from build123d import *

# Parameters (mm, degrees)
F0_W      = 6.35
F0_H      = 6.35
F1_DEPTH  = 3.81
F2_R      = 2.3894248051
F3_DEPTH  = 25.4
F8_R      = 0.2232162281
F9_DEPTH  = 25.4
F10_R     = 2.7317429941
F11_DEPTH = 3.4770822
F12_W     = 5.8086237404
F12_H     = 6.0867127031
F13_DEPTH = 25.4


with BuildPart() as f1:
    # F0 (on Top) → F1 (new body)
    with BuildSketch(Plane.XY):
        with Locations((2.5444868952, -10.8615327454)):
            Rectangle(F0_W, F0_H)
    extrude(amount=F1_DEPTH)

    # F2 (on face) → F3 (join)
    with BuildSketch(Plane.XY.offset(3.81)):
        with Locations((2.5444868952, -10.8615327454)):
            Circle(F2_R)
    extrude(amount=F3_DEPTH)


with BuildPart() as f1_1:
    # F4: moved
    add(f1.part.moved(Location((-2.4892, 10.8204, 0))))

    # F5 (on Front) → F6 (revolve)
    with BuildSketch(Plane.XZ):
        with BuildLine():
            Line((3.715344239, 29.1360206902), (2.3982734419, 29.1360206902))
            Line((2.3982734419, 29.1360206902), (2.3982734419, 25.658948347))
            Line((2.3982734419, 25.658948347), (3.715344239, 25.658948347))
            ThreePointArc((3.715344239, 25.658948347), (3.8481047551, 26.626173701), (4.5479801483, 27.3068532688))
            Line((4.5479801483, 27.3068532688), (4.5479801483, 29.1360206902))
            Line((4.5479801483, 29.1360206902), (3.715344239, 29.1360206902))
        make_face()
    revolve(axis=Axis((0.0552868952, -0.0411327454, 29.21), (0, 0, 1)))


with BuildPart() as f1_2:
    # F7: moved
    add(f1_1.part.moved(Location((-0.0508, 0.0508, 0))))

    # F8 (on face) → F9 (cut)
    with BuildSketch(Plane.XY.offset(29.21)):
        with BuildLine():
            ThreePointArc((0.2196997185, 2.5085243013), (-0.06466925, 2.7232003988), (-0.1932256967, 2.3908981612))
            ThreePointArc((-0.1932256967, 2.3908981612), (-0.0028015905, 2.2853092181), (0.1869422498, 2.3921157731))
            ThreePointArc((0.1869422498, 2.3921157731), (0.2113543474, 2.4480594413), (0.2196997185, 2.5085243013))
        make_face()
        with Locations((-1.4773185054, 2.027371838)):
            Circle(F8_R)
        with Locations((-2.3868350443, 0.7718322405)):
            Circle(F8_R)
        with Locations((-2.3846617218, -0.7785210393)):
            Circle(F8_R)
        with Locations((-1.4716286733, -2.031505743)):
            Circle(F8_R)
        with Locations((0.0035165096, -2.5085243013)):
            Circle(F8_R)
        with Locations((1.4773185054, -2.027371838)):
            Circle(F8_R)
        with Locations((2.3868350443, -0.7718322405)):
            Circle(F8_R)
        with Locations((2.3846617218, 0.7785210393)):
            Circle(F8_R)
        with Locations((1.4716286733, 2.031505743)):
            Circle(F8_R)
    extrude(amount=-F9_DEPTH, mode=Mode.SUBTRACT)

    # F10 (on face) → F11 (join)
    with BuildSketch(Plane.XY.offset(29.1360206902)):
        Circle(F10_R)
    extrude(amount=-F11_DEPTH)

    # F12 (on face) → F13 (cut)
    with BuildSketch(Plane.XY.offset(29.1360206902)):
        with Locations((0.0104332576, 0.1239965204)):
            Rectangle(F12_W, F12_H)
    extrude(amount=F13_DEPTH, mode=Mode.SUBTRACT)


solid = f1_2.part
Model file for the job. Use its own axes, mm. A direction names the side the tool comes from. Round coordinates to 2 decimals unless told otherwise and drop trailing zeros. Loops run counter-clockwise (first coordinate to the right, second up) from the corner with the lowest first, then second, coordinate; pieces in that order, holes last. Notation, with made-up numbers: (15.5, 75.25) - (62.5, 75.25) arc R15 cw to (62.5, 93.25) - close; hole circle Ø4 at (-20.75, 81). An arc over 180 degrees is marked (long way). Write each question's results on one line, items separated by ' | '.
(1) Saw through at B-B, the plane z = 3. List the corners of the cut face in (x, y), then the cut area to 3 significant figures.
Answer below:
outline: (-3.17, -3.17) - (3.18, -3.17) - (3.18, 3.18) - (-3.17, 3.18) - close | area: 40.3 mm^2
(2) Wall check: L1, parallel to Z at x = -2.75, y = 1.5; L2, parallel to Y at x = -1.5, z = 8.75; L3, parallel to Y at x = -0.25, z = 10.5. Give the ranges that are in metal, low to high.
Answer below:
L1: z = 0 to 3.81, 25.66 to 29.14 | L2: y = -1.81 to 1.81 | L3: y = -2.37 to 2.39
(3) Mould opens along Z. For faces 6 (the cylindrical face through (-0.74, -2.26, 14.58)), 7 (the flat face through (-3.171, 0, 2)), 8 (the flat face through (0, 0, 0)) say: released by +Z, released by -Z, zero draft, split by the parting line, or undercut.
Answer below:
face 6: undercut | face 7: zero draft | face 8: released by -Z
(4) Pin check, flat tips, straight feed: pin 1 (1.1 mm diameter, centred on x = 1, z = 3, fed in from +Y); pin 2 (2 mm diameter, centred on x = -3, z = 18.5, fed in from -Y); pin 3 (5 mm diameter, centred on x = 2, z = 15, fed in from -Y). Stop position of each tip, or through.
Answer below:
pin 1: stops at y = 3.18 | pin 2: stops at y = -1.29 | pin 3: stops at y = -2.37
(5) 3-axis set-ups, long thin cutter, end or side, ignore diameter. For faces 1 (the cylindrical face through (0.75, 2.28, 14.58)), 2 (the cylindrical face through (0.731, -2.267, 14.582)), 3 (the flat face through (0, -3.165, 2)), 4 (the flat face through (-1.5, 2.2, 3.81)), 5 (the cylindrical face through (-1.928, -1.396, 14.582)): which of +Z, -Z, +X, -X, +Y, -Y reach the whole face in a straight line?
Answer below:
face 1: +X, +Y | face 2: +X, -Y | face 3: -Z, +X, -X, -Y | face 4: none | face 5: -X, -Y
(6) Saw through at A-A, the plane z = 14. List the corners of the cut face in (x, y), then the cut area to 3 significant figures.
Answer below:
outline: (-2.32, 0.56) arc R2.39 ccw to (-2.31, -0.57) arc R0.22 cw to (-2.2, -0.91) arc R2.39 ccw to (-1.54, -1.82) arc R0.22 cw to (-1.25, -2.02) arc R2.39 ccw to (-0.17, -2.37) arc R0.22 cw to (0.18, -2.37) arc R2.39 ccw to (1.25, -2.03) arc R0.22 cw to (1.55, -1.82) arc R2.39 ccw to (2.21, -0.91) arc R0.22 cw to (2.33, -0.56) arc R2.39 ccw to (2.33, 0.56) arc R0.22 cw to (2.21, 0.92) arc R2.39 ccw to (1.56, 1.83) arc R0.22 cw to (1.25, 2.05) arc R2.39 ccw to (0.19, 2.39) arc R0.22 cw to (-0.19, 2.39) arc R2.39 ccw to (-1.25, 2.04) arc R0.22 cw to (-1.56, 1.82) arc R2.39 ccw to (-2.21, 0.91) arc R0.22 cw to start | area: 17.7 mm^2
